```python
from build123d import *

# Parameters (mm, degrees)
SKETCH1_R           = 3.175
SKETCH1_R_2         = 1.5875
BOSS_EXTRUDE1_DEPTH = 3.048


with BuildPart() as part:
    # Sketch1 → Boss-Extrude1 (new, symmetric)
    with BuildSketch(Plane(origin=(0, 0, 0), x_dir=(1, 0, 0), z_dir=(0, 1, 0))):
        with BuildLine():
            Line((-9.099235244, -0.903689094), (-3.807571336, -54.185393016))
            ThreePointArc((-3.807571336, -54.185393016), (14.328591511, -92.658850534), (52.678421921, -111.054987185))
            ThreePointArc((52.678421921, -111.054987185), (58.779230265, -108.583775292), (60.117170229, -102.138880621))
            ThreePointArc((60.117170229, -102.138880621), (60.633172254, -94.28427436), (66.105273821, -88.625899853))
            ThreePointArc((66.105273821, -88.625899853), (71.266071099, -80.525710338), (66.339661954, -72.280870032))
            ThreePointArc((66.339661954, -72.280870032), (50.960508132, -62.625906994), (37.347898209, -50.607856626))
            Line((37.347898209, -50.607856626), (29.464, -50.607856626))
            Line((29.464, -50.607856626), (29.464, -41.476271417))
            ThreePointArc((29.464, -41.476271417), (16.820103433, -20.840439396), (8.915029824, 2.033464836))
            ThreePointArc((8.915029824, 2.033464836), (-1.47146227, 9.024828796), (-9.099235244, -0.903689094))
        make_face()
        Circle(SKETCH1_R, mode=Mode.SUBTRACT)
        with Locations((62.123011123, -80.394598631)):
            Circle(SKETCH1_R, mode=Mode.SUBTRACT)
        with Locations((54.567235003, -104.644758367)):
            Circle(SKETCH1_R, mode=Mode.SUBTRACT)
        with Locations((10.16, -40.64)):
            Circle(SKETCH1_R_2, mode=Mode.SUBTRACT)
        with Locations((20.32, -81.28)):
            Circle(SKETCH1_R_2, mode=Mode.SUBTRACT)
    extrude(amount=BOSS_EXTRUDE1_DEPTH, both=True)


solid = part.part
```
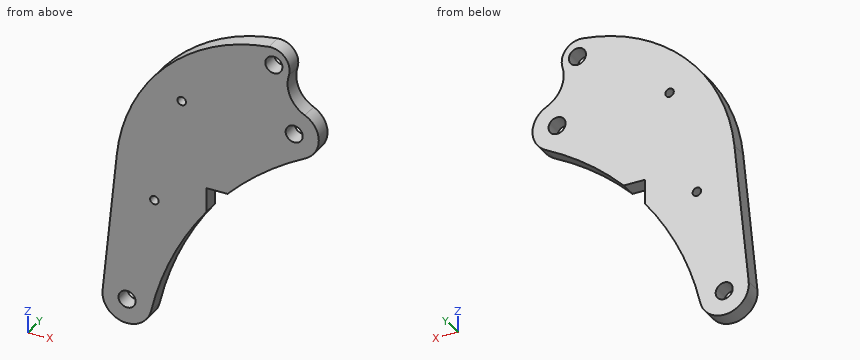
Geometry: final body of the model. Coordinates: model frame, mm. Round coordinates to 2 decimals unless told otherwise and drop trailing zeros. Order: outer loops, then holes, each group sorted by start corner. A loop starts at its lowest first (then second) coordinate and runs counter-clockwise, first axis right, second up. Notation, with made-up numbers: (74, 79) - (97, 79) arc R4 ccw to (97, 83) - close; hole circle Ø10 at (36, 84.25). An arc over 180 degrees is marked (long way). Use CSV: the item, a comma, the result in double quotes. Start each with the question number.
Q1. Section query C-C (x = 0). Return loops of the section in (y, z) (3 decimals).
Q2. Material intervals for line 1 along X through (y, z) = (-1.5, 81.28); line 2 along X through (y, z) = (1.25, 0) (3 decimals); line 3 along Z through (x, y) = (21.5, -2.25), sorted ascending. Write a range as from..to.
Q3. Section query D-D (z = 68). Return loops of the section in (x, y), and give its area (3 significant figures).
Q4. Section query B-B (y = -1.5). State how many separate pieces and enclosed holes the cut face has, and give its area (3 significant figures).
Q5. Section query A-A (x = 10.16). Return loops of the section in (y, z).
Q6. First-contact query: pin 1 (2 mm diameter, centred on x = 63, y = 0, fed in from +Z); pin 2 (2 mm diameter, centred on y = 1.5, z = 73.5, fed in from +X); pin 3 (1.9 mm diameter, centred on x = 10.16, z = 40.64, fed in from +Y); pin 4 (1.8 mm diameter, centred on y = 1, z = 46.5, fed in from +X). Flat tips, straight axial feed; report the tip coordinate or a pass-through.
Result set:
1,outline,"(-3.048, -9.144) - (3.048, -9.144) - (3.048, -3.175) - (-3.048, -3.175) - close; (-3.048, 3.175) - (3.048, 3.175) - (3.048, 70.406) - (-3.048, 70.406) - close"
2,line 1,"x = 5.36..18.73, 21.91..59.07, 65.17..71.22"
2,line 2,"x = -9.144..-3.175, 3.175..9.399"
2,line 3,"z = 29.7..80.22, 82.34..98.87"
3,outline,"(-0.86, -3.05) - (58.83, -3.05) - (58.83, 3.05) - (-0.86, 3.05) - close"
3,area,"364 mm2"
4,separate pieces,"1"
4,enclosed holes,"5"
4,area,"4,350 mm2"
5,outline,"(-3.05, 2.9) - (3.05, 2.9) - (3.05, 39.05) - (-3.05, 39.05) - close; (-3.05, 42.23) - (3.05, 42.23) - (3.05, 88.03) - (-3.05, 88.03) - close"
6,pin 1,"stops at z = 91.98"
6,pin 2,"stops at x = 69.11"
6,pin 3,"passes through"
6,pin 4,"stops at x = 29.46"
